Source: CAD feature listing. Evaluate the final solid. Frame: model axes, mm. A direction names the side the tool comes from. Give positions to 0.01 mm unless a question says otherwise; leave off trailing zeros. Order: outer loops, then holes, each group sorted by start corner. A loop starts at its lowest first (then second) coordinate and runs counter-clockwise, first axis right, second up. Notation, with made-up numbers: (45, -31) - (72, -31) arc R26 ccw to (72, -16) - close; hole circle Ø3 at (40, 18). An arc over 180 degrees is marked (long way). Use CSV: the item, a comma, the result in double quotes.
Autodesk Inventor part; units mm, degrees
ref_plane "YZ Plane" through (0, 0, 0) normal (1, 0, 0) x (0, 1, 0)
ref_plane "XZ Plane" through (0, 0, 0) normal (0, 1, 0) x (-1, 0, 0)
ref_plane "XY Plane" through (0, 0, 0) normal (0, 0, 1) x (1, 0, 0)
sketch "Boceto1" plane through (0, 0, 0) normal (0, 1, 0) x (-1, 0, 0)
  line L0 (100, 100) -> (-100, 100)
  line L1 (-100, 100) -> (-100, -100)
  line L2 (-100, -100) -> (100, -100)
  line L3 (100, -100) -> (100, 100)
  line L4 (100, 100) -> (-100, -100) construction
  line L5 (-100, 100) -> (100, -100) construction
  point P0 (0, 0)
  dimension "d0" = 200
  dimension "d1" = 200
extrude "Extrusión1" add sketch "Boceto1" along normal blind 20
sketch "Boceto2" plane through (0, 20, 0) normal (0, 1, 0) x (1, 0, 0)
  circle A0 centre (-11.5239, -30.0616) radius 3
  circle A1 centre (11.4761, -30.0616) radius 3
  circle A2 centre (-11.5239, -60.0616) radius 3
  circle A3 centre (11.4761, -60.0616) radius 3
  line L0 (-0.0239, -45.0616) -> (-35.0239, -45.0616)
  line L1 (-35.0239, -45.0616) -> (-35.0239, -80.0616)
  line L2 (-0.0239, -45.0616) -> (34.9761, -45.0616)
  line L3 (-11.5239, -30.0616) -> (11.4761, -60.0616)
  line L4 (-11.5239, -60.0616) -> (11.4761, -30.0616)
  line L5 (34.9761, -20.0616) -> (-35.0239, -20.0616)
  line L6 (-35.0239, -20.0616) -> (-35.0239, -80.0616)
  line L7 (34.9761, -80.0616) -> (34.9761, -20.0616)
  line L8 (-105, -100.0616) -> (105, -100.0616)
  line L9 (-105.0239, -80.0616) -> (104.9761, -80.0616)
  line L10 (-35.0239, -80.0616) -> (34.9761, -80.0616)
  line L11 (105, -100.0616) -> (95.8154, -100.0616)
  line L12 (-105.0239, -80.0616) -> (104.9761, -80.0616)
  line L13 (105, -80.0616) -> (-105, -80.0616)
  line L14 (-105, -100.0616) -> (105, -100.0616)
  line L15 (105, -90.0616) -> (94.0798, -90.0616)
  line L16 (-105, -100.0616) -> (105, -100.0616)
  line L17 (-105, -80.0616) -> (105, -80.0616)
  line L18 (105, -80.0616) -> (105, -100.0616)
  line L19 (105, -100.0616) -> (-105, -100.0616)
  line L20 (-105, -100.0616) -> (-105, -80.0616)
  line L21 (-100, 100) -> (-100, -100)
  line L22 (-100, -100) -> (100.4077, -100)
  point P0 (0, 0)
  point P1 (0, -10.0616)
  point P2 (0, -90.0616)
  point P3 (-0.0478, -80.0616)
  dimension "d4" = 20
  dimension "d5" = 20
  dimension "d6" = 30
  dimension "d7" = 30
  dimension "d8" = 20
  dimension "d9" = 35
  dimension "d10" = 35
  dimension "d11" = 60
extrude "Extrusión2" cut sketch "Boceto2" against normal blind 10
sketch "Boceto3" plane through (0, 20, 0) normal (0, 1, 0) x (1, 0, 0)
  circle A0 centre (-11.5239, -30.0616) radius 3
  circle A1 centre (-11.5239, -30.0616) radius 3
  circle A2 centre (11.4761, -30.0616) radius 3
  circle A3 centre (11.4761, -30.0616) radius 3
  circle A4 centre (11.4761, -60.0616) radius 3
  circle A5 centre (11.4761, -60.0616) radius 3
  circle A6 centre (-11.5239, -60.0616) radius 3
  point P0 (0, 0)
extrude "Extrusión3" cut sketch "Boceto3" against normal blind 20
sketch "Boceto4" plane through (0, 20, 0) normal (0, 1, 0) x (1, 0, 0)
  circle A0 centre (-51.75, 78.25) radius 1.75
  line L0 (-50, 70) -> (-60, 70)
  line L1 (-60, 70) -> (-60, 80)
  line L2 (-60, 80) -> (-50, 80)
  line L3 (-50, 80) -> (-50, 70)
  line L4 (-50, 70) -> (-60, 80) construction
  line L5 (-60, 70) -> (-50, 80) construction
  line L6 (-105, 90) -> (-105, -90)
  circle A1 centre (-58.25, 71.75) radius 1.75
  line L7 (0, 90) -> (0, 77.3124)
  circle A2 centre (51.75, 78.25) radius 1.75
  line L8 (50, 70) -> (60, 70)
  line L9 (60, 70) -> (60, 80)
  line L10 (60, 80) -> (50, 80)
  line L11 (50, 80) -> (50, 70)
  line L12 (50, 70) -> (60, 80) construction
  line L13 (60, 70) -> (50, 80) construction
  circle A3 centre (58.25, 71.75) radius 1.75
  line L14 (100, 100) -> (-100, 100)
  line L15 (-100, 100) -> (-100, -80.0616)
  line L16 (100, -80.0616) -> (100, 100)
  point P0 (0, 0)
  point P1 (0, 0)
  point P2 (-60, 75)
  point P3 (60, 75)
  dimension "d16" = 3.5
  dimension "d18" = 1.75
  dimension "d19" = 1.75
  dimension "d20" = 1.75
  dimension "d21" = 1.75
  dimension "d22" = 10
  dimension "d23" = 10
  dimension "d25" = 20
  dimension "d26" = 40
  dimension "d27" = 40
hole "Agujero1" at (-58.25, 20, -71.75) at (-51.75, 20, -78.25) at (58.25, 20, -71.75) at (51.75, 20, -78.25) direction (0, -1, 0) diameter 3.5 end through all
sketch "Boceto5" plane through (0, 20, 0) normal (0, 1, 0) x (1, 0, 0)
  line L0 (0, 90) -> (0, 68.25)
  circle A0 centre (-51.75, 78.25) radius 1.75
  line L1 (-50, 78.25) -> (-50, 100)
  circle A1 centre (-58.25, 71.75) radius 1.75
  line L2 (-60, 71.75) -> (-60, 100)
  line L3 (-60, 100) -> (-70, 100)
  line L4 (-50, 100) -> (-40, 100)
  line L5 (-40, 100) -> (-40, 60)
  line L6 (-40, 60) -> (-70, 60)
  line L7 (-70, 60) -> (-70, 100)
  line L8 (-70, 100) -> (-40, 100)
  circle A2 centre (51.75, 78.25) radius 1.75
  line L9 (50, 78.25) -> (50, 100)
  circle A3 centre (58.25, 71.75) radius 1.75
  line L10 (60, 71.75) -> (60, 100)
  line L11 (60, 100) -> (70, 100)
  line L12 (50, 100) -> (40, 100)
  line L13 (40, 100) -> (40, 60)
  line L14 (40, 60) -> (70, 60)
  line L15 (70, 60) -> (70, 100)
  line L16 (70, 100) -> (40, 100)
  point P0 (0, 0)
  dimension "d38" = 10
  dimension "d39" = 10
  dimension "d40" = 40
extrude "Extrusión4" cut sketch "Boceto5" against normal blind 10
ref_plane "Plano de trabajo1" through (0, 0, -100) normal (-1, 0, 0) x (0, 0, 1)
ref_plane "Plano de trabajo2" through (100, 0, 0) normal (0, 0, -1) x (-1, 0, 0)
sketch "Boceto7" plane through (0, 0, 0) normal (0, -1, 0) x (1, 0, 0)
  circle A0 centre (10, -10) radius 1.75
  line L0 (6.803, 0) -> (14.6069, 0)
  line L1 (0, 0) -> (0, -4.8284)
  line L2 (0, 0) -> (20.0354, 0)
  circle A1 centre (10, 10) radius 1.75
  line L3 (0, 0) -> (0, 4.8284)
  circle A2 centre (-10, -10) radius 1.75
  circle A3 centre (-10, 10) radius 1.75
  dimension "d52" = 3.5
  dimension "d54" = 10
  dimension "d55" = 10
hole "Agujero2" at (10, 0, -10) at (10, 0, 10) at (-10, 0, 10) at (-10, 0, -10) direction (0, 1, 0) diameter 3.5 end through all
sketch "Boceto8" plane through (0, 0, 0) normal (0, -1, 0) x (1, 0, 0)
  line L0 (-15, 15) -> (15, 15)
  line L1 (15, 15) -> (15, -15)
  line L2 (15, -15) -> (-15, -15)
  line L3 (-15, -15) -> (-15, 15)
  line L4 (-15, 15) -> (15, -15) construction
  line L5 (15, 15) -> (-15, -15) construction
  point P0 (0, 0)
  dimension "d63" = 30
  dimension "d64" = 30
extrude "Extrusión5" cut sketch "Boceto8" against normal blind 10
sketch "Boceto9" plane through (0, 0, 0) normal (0, -1, 0) x (1, 0, 0)
  circle A0 centre (85, -10) radius 1.75
  line L0 (100, 100) -> (100, -100)
  line L1 (140, 0) -> (-140, 0)
  circle A1 centre (85, 10) radius 1.75
  line L2 (0, 0) -> (0, 9.4908)
  circle A2 centre (-85, -10) radius 1.75
  circle A3 centre (-85, 10) radius 1.75
  line L3 (0, 0) -> (6.3157, 6.3157)
  line L4 (0, 0) -> (8.9318, 0) construction
  circle A4 centre (10, 85) radius 1.75
  circle A5 centre (-10, -85) radius 1.75
  line L5 (0, 0) -> (5.9531, -5.9531)
  line L6 (0, 0) -> (8.419, 0) construction
  circle A6 centre (10, -85) radius 1.75
  circle A7 centre (-10, 85) radius 1.75
  dimension "d67" = 3.5
  dimension "d68" = 15
  dimension "d69" = 10
  dimension "d70" = 45
  dimension "d71" = 45
hole "Agujero3" at (-10, 0, 85) at (10, 0, 85) at (85, 0, 10) at (85, 0, -10) at (-85, 0, 10) at (-85, 0, -10) at (-10, 0, -85) at (10, 0, -85) direction (0, 1, 0) diameter 3.5 end through all
split "Dividir3" plane through (100, 0, 0) removes the side toward (0, 0, 1)
split "Dividir4" plane through (0, 0, -100) removes the side toward (-1, 0, 0)
properties part number "base_front_2"
Item 1: Section C-C on y = 4.5. Return the cut outline in (x, z), then the cut area to 3 significant figures.
Filled in:
outline,"(0, -100) - (100, -100) - (100, 0) - (15, 0) - (15, -15) - (0, -15) - close; hole circle Ø3.5 at (10, -85); hole circle Ø3.5 at (51.75, -78.25); hole circle Ø3.5 at (58.25, -71.75); hole circle Ø3.5 at (85, -10)"
area,"9,740 mm2"
Item 2: Section A-A on z = -71.75. Return the cut outline in (x, y), then the cut area to 4 significant figures.
Filled in:
outline,"(0, 0) - (56.5, 0) - (56.5, 10) - (40, 10) - (40, 20) - (0, 20) - close; (60, 0) - (100, 0) - (100, 20) - (70, 20) - (70, 10) - (60, 10) - close"
area,"1,665 mm2"
Item 3: Material intervals for line 1 (Z direction, x = 10, y = 8); line 2 (Z direction, x = 85, y = 5.5); line 3 (X direction, y = 14.5, z = -81.5), sorted ascending. Write a range as from..to.
Filled in:
line 1,"z = -100..-86.75, -83.25..-15"
line 2,"z = -100..-11.75, -8.25..0"
line 3,"x = 0..40, 70..100"
Item 4: Section D-D on x = 58.25. Return the cut outline in (y, z), then the cut area to 4 significant figures.
Filled in:
outline,"(0, -100) - (10, -100) - (10, -73.5) - (0, -73.5) - close; (0, -70) - (10, -70) - (10, -60) - (20, -60) - (20, 0) - (0, 0) - close"
area,"1,565 mm2"
Item 5: Set-up query: faces 5 (the flat face through (70, 15, -80)), 6 (the flat face through (8, 5, -15)), 7 (the flat face through (51, 0, -49)). Return all of +Z, -Z, +X, -X, +Y, -Y with unobstructed straight access to the full face (end or side cutting, diameter ignored); none if empty.
Filled in:
face 5,"-Z, +Y"
face 6,"+Z, -X, -Y"
face 7,"+Z, -Z, +X, -X, -Y"
Item 6: First-contact query: pin 1 (3 mm diameter, centred on x = 58, y = 14.5, fed in from -Z); pin 2 (9 mm diameter, centred on x = 52, z = -89.5, fed in from +Y); pin 3 (1.5 mm diameter, centred on x = 11, y = 6.5, fed in from +Z); pin 4 (2 mm diameter, centred on x = 10, z = -10, fed in from -Y). Flat tips, straight axial feed; report the tip coordinate or a pass-through.
Filled in:
pin 1,"stops at z = -60"
pin 2,"stops at y = 10"
pin 3,"stops at z = -15"
pin 4,"passes through"
Item 7: Section B-B on x = 10. Return the cut outline in (y, z).
Filled in:
outline,"(0, -100) - (20, -100) - (20, -86.75) - (0, -86.75) - close; (0, -83.25) - (20, -83.25) - (20, -11.75) - (10, -11.75) - (10, -15) - (0, -15) - close; (10, -8.25) - (20, -8.25) - (20, 0) - (10, 0) - close"
Item 8: Mould query, pull axis X, two halves, no side actions, for faces 1 (the flat face through (7, 10, -7)), 2 (the flat face through (100, 10, -49)), 3 (the flat face through (40, 15, -80)), 4 (the cylindrical face through (8.5, 15.1, -10.9)). Classes: released by +X, released by -X, zero draft, split by the parting line, or undercut.
Filled in:
face 1,"zero draft"
face 2,"released by +X"
face 3,"undercut"
face 4,"undercut"
